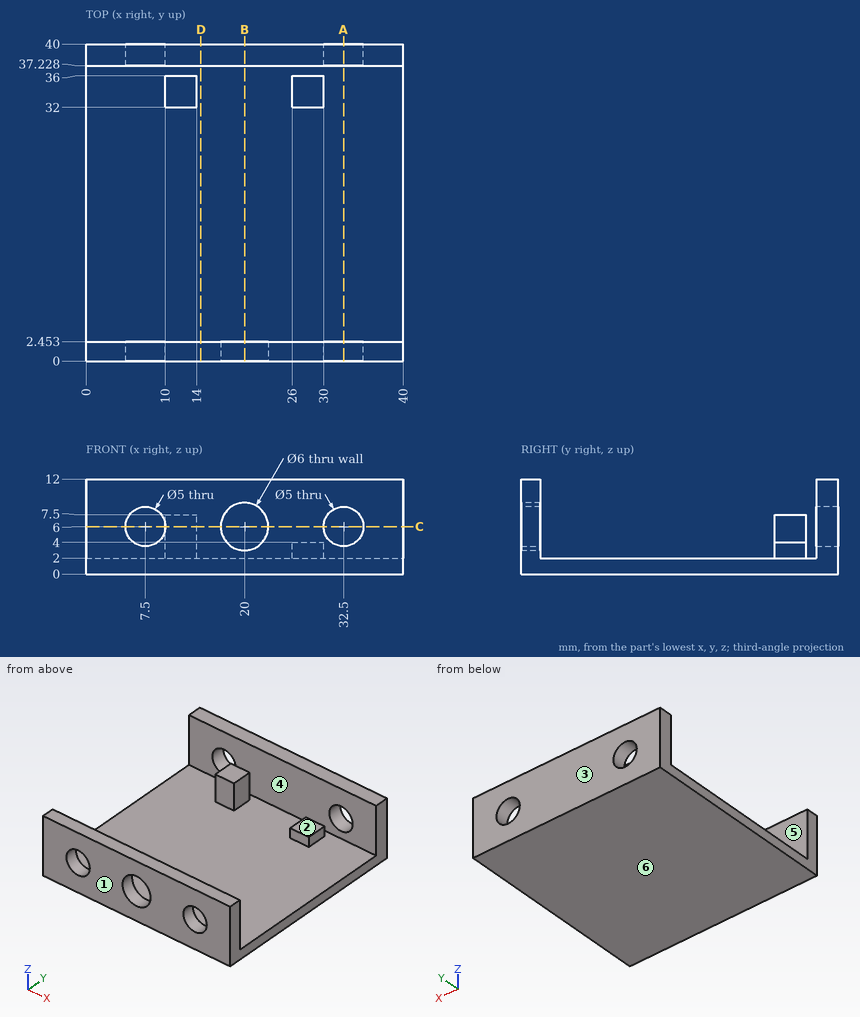
Print and shaded views of the part. All mm, measured from the part's lowest x, y and z. A direction names the side the tool comes from. Round coordinates to 2 decimals unless told otherwise and drop trailing zeros. Write each loop counter-clockwise with the first axis right and the second up, starting at its lowest first coordinate (ties: lowest second). Pieces come first, ordered by that corner, then holes. Notation, with made-up numbers: (62, -17.75) -> (69, -17.75) arc R20 cw to (69, 17.25) -> close; hole circle Ø1 at (55, 55). An arc over 180 degrees is marked (long way). Return JSON: item names as keys, results as strings. Group by question number.
Q1. Saw through at D-D on x = 14.5. Write the cut outline in (y, z), plus the area to 3 significant figures.
Q2. Mould opens along Y. For the marked faces 1, 2, 3 and 4 say: pulls with the +Y half, pulls with the -Y half, needs draft (parallel to the pull), parting line crosses it, or undercut.
Q3. Pin check, flat tips, straight feed: pin 1 (1 mm diameter, centred on x = 27.5, z = 3, fed in from -Y); pin 2 (1 mm diameter, centred on y = 34, z = 3, fed in from +X); pin 3 (1.2 mm diameter, centred on x = 12, y = 34, fed in from +Z). Stop position of each tip, or through.
Q4. Which spindle directions (+Z, -Z, +X, -X, +Y, -Y) get a long thin tool onto all of the face, cutting with end or side? Do the marked faces 5 and 6. Say none if no direction does.
Q5. Saw through at A-A on x = 32.5. Write the cut outline in (y, z), plus the area to 3 significant figures.
Q6. Saw through at C-C on z = 6. State how many separate pieces and enclosed holes the cut face has, plus the area to 3 significant figures.
Q7. Saw through at B-B on x = 20. Write the cut outline in (y, z).
Q8. Probe L1, parallel to X at y = 1.8, z = 6; L2, parallel to Y at x = 2.5, z = 3; L3, parallel to X at y = 39.1, z = 6. List the from-to ranges inside material, lowest first. Write a range as [from, to].
Answer:
{
 "1": {"outline": "(0, 0) -> (40, 0) -> (40, 12) -> (37.23, 12) -> (37.23, 2) -> (2.45, 2) -> (2.45, 12) -> (0, 12) -> close", "area": "132 mm2"},
 "2": {"face 1": "pulls with the -Y half", "face 2": "undercut", "face 3": "pulls with the +Y half", "face 4": "undercut"},
 "3": {"pin 1": "y = 0", "pin 2": "x = 30", "pin 3": "z = 7.5"},
 "4": {"face 5": "+Z, +X, -X", "face 6": "-Z, +X, -X, +Y, -Y"},
 "5": {"outline": "(0, 0) -> (40, 0) -> (40, 3.5) -> (37.23, 3.5) -> (37.23, 2) -> (2.45, 2) -> (2.45, 3.5) -> (0, 3.5) -> close; (0, 8.5) -> (2.45, 8.5) -> (2.45, 12) -> (0, 12) -> close; (37.23, 8.5) -> (40, 8.5) -> (40, 12) -> (37.23, 12) -> close", "area": "106 mm2"},
 "6": {"separate pieces": "8", "enclosed holes": "0", "area": "158 mm2"},
 "7": {"outline": "(0, 0) -> (40, 0) -> (40, 12) -> (37.23, 12) -> (37.23, 2) -> (2.45, 2) -> (2.45, 3) -> (0, 3) -> close; (0, 9) -> (2.45, 9) -> (2.45, 12) -> (0, 12) -> close"},
 "8": {"L1": "[0, 5], [10, 17], [23, 30], [35, 40]", "L2": "[0, 2.45], [37.23, 40]", "L3": "[0, 5], [10, 30], [35, 40]"}
}
